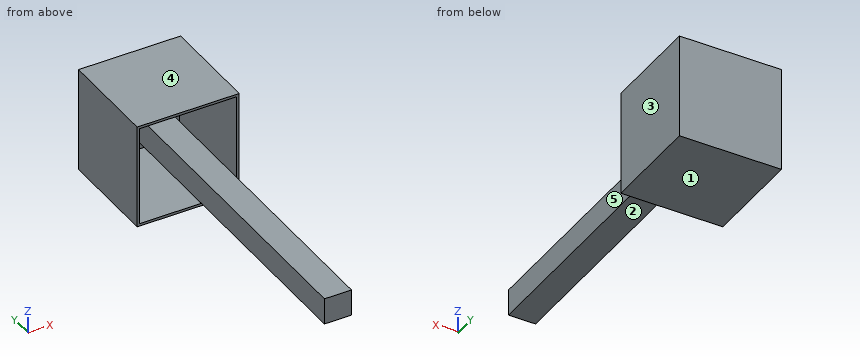
from build123d import *

# Parameters (mm, degrees)
F0_W     = 102.5334298611
F0_H     = 105.3606420755
F1_DEPTH = 50.8
F2_T     = -2.54
F3_W     = 27.1412022412
F3_H     = 26.5757590532
F4_DEPTH = 48.26
F5_DEPTH = 310.35808


with BuildPart() as f1:
    # F0 (on Front) → F1 (new body, symmetric)
    with BuildSketch(Plane.XZ):
        Rectangle(F0_W, F0_H)
    extrude(amount=F1_DEPTH, both=True)

    # F2
    f2_openings = [f1.faces().sort_by_distance(p)[0] for p in [
        (0, -50.8, 0),
    ]]
    offset(amount=F2_T, openings=f2_openings)

    # F3 (on Front) → F4 (join, through all)
    with BuildSketch(Plane.XZ):
        Rectangle(F3_W, F3_H)
    extrude(amount=-F4_DEPTH)

    # F5 (add): a face of the model
    f5_faces = [f1.faces().sort_by_distance(p)[0] for p in [
        (0, 0, 0),
    ]]
    extrude(f5_faces, amount=F5_DEPTH)


solid = f1.part
The listing builds one solid part. Answer for the finished solid, in the listing's coordinates (mm). Face numbers are marked on the shaded views. A direction names the side the tool comes from. Coordinates: 2 decimals unless noted, no trailing zeros. Loops run counter-clockwise (first coordinate to the right, second up) from the corner with the lowest first, then second, coordinate; pieces in that order, holes last. Notation, with made-up numbers: (-6, -11.5) -> (27, -11.5) arc R29 cw to (27, 26.5) -> close; hole circle Ø11 at (-6.5, 34.5). An arc over 180 degrees is marked (long way). Answer in a Markdown table with one row per item. Add a question column.
1. The part is cut by section C-C, the plane z = 4. Write down the section's boundary in (x, y).
2. The part is cut by section A-A, the plane y = 18. Write down the section's boundary in (x, z), then the cut area to 3 significant figures.
3. Consider line 1 (X direction, y = -50.5, z = 12.5); line 2 (X direction, y = -30.5, z = 14); line 3 (Z direction, x = 41.5, y = 14). Determine where each line is inside the solid, lowest interval first. Write a range as [from, to].
4. The part is cut by section D-D, the plane z = -26. Write down the section's boundary in (x, y), then the cut area to 3 significant figures.
5. For the marked faces 4 and 5, determine the directions among +Z, -Z, +X, -X, +Y, -Y from which every point of the face is accessible in a straight line to the end or side of a thin tool.
6. Flat-ended cylindrical pins translate along their axes: P1, Ø3, axis at y = -82.5, z = -11.5, coming from the +X side; P2, Ø8, axis at x = 3, y = -214, coming from the -Z side; P3, Ø13.5, axis at x = 5.5, y = -156, coming from the +Z side. Find the tip coordinate at first contact, or state that the pin passes through.
7. Determine the mould class of the marked faces 1, 2 and 3 for opening direction X: +X half, -X half, draft (parallel to the pull), parting line (faces both ways), or undercut.
8. The part is cut by section B-B, the plane x = -10. Write down the section's boundary in (y, z), then the cut area to 3 significant figures.
Answer below:
| question | item | result |
|---|---|---|
| 1 | outline | (-51.27, -50.8) -> (-48.73, -50.8) -> (-48.73, 48.26) -> (-13.57, 48.26) -> (-13.57, -310.36) -> (13.57, -310.36) -> (13.57, 48.26) -> (48.73, 48.26) -> (48.73, -50.8) -> (51.27, -50.8) -> (51.27, 50.8) -> (-51.27, 50.8) -> close |
| 2 | outline | (-51.27, -52.68) -> (51.27, -52.68) -> (51.27, 52.68) -> (-51.27, 52.68) -> close; (-13.57, -13.29) -> (13.57, -13.29) -> (13.57, 13.29) -> (-13.57, 13.29) -> close; hole (-48.73, -50.14) -> (48.73, -50.14) -> (48.73, 50.14) -> (-48.73, 50.14) -> close |
| 2 | area | 1,750 mm2 |
| 3 | line 1 | [-51.27, -48.73], [-13.57, 13.57], [48.73, 51.27] |
| 3 | line 2 | [-51.27, -48.73], [48.73, 51.27] |
| 3 | line 3 | [-52.68, -50.14], [50.14, 52.68] |
| 4 | outline | (-51.27, -50.8) -> (-48.73, -50.8) -> (-48.73, 48.26) -> (48.73, 48.26) -> (48.73, -50.8) -> (51.27, -50.8) -> (51.27, 50.8) -> (-51.27, 50.8) -> close |
| 4 | area | 764 mm2 |
| 5 | face 4 | +Z, +X, -X, +Y, -Y |
| 5 | face 5 | -Y |
| 6 | P1 | x = 13.57 |
| 6 | P2 | z = -13.29 |
| 6 | P3 | z = 13.29 |
| 7 | face 1 | draft |
| 7 | face 2 | undercut |
| 7 | face 3 | +X half |
| 8 | outline | (-310.36, -13.29) -> (48.26, -13.29) -> (48.26, -50.14) -> (-50.8, -50.14) -> (-50.8, -52.68) -> (50.8, -52.68) -> (50.8, 52.68) -> (-50.8, 52.68) -> (-50.8, 50.14) -> (48.26, 50.14) -> (48.26, 13.29) -> (-310.36, 13.29) -> close |
| 8 | area | 10,300 mm2 |
